Build history of the part. All positions in model axes, mm. A direction names the side the tool comes from. Give positions to 0.01 mm unless a question says otherwise; leave off trailing zeros. Write each loop counter-clockwise with the first axis right and the second up, starting at its lowest first coordinate (ties: lowest second). Pieces come first, ordered by that corner, then holes. Notation, with made-up numbers: (8.5, 81.5) -> (12.5, 81.5) arc R25 cw to (12.5, 100.5) -> close; hole circle Ø3 at (40, 64.5). An arc over 180 degrees is marked (long way). Put each result on its own line as item: value. Start each with the question number.
Item 1: Drill centre lines: line 1 along X through (y, z) = (-3.2, 5); line 2 along Z through (x, y) = (0, -6); line 3 along X through (y, z) = (-4, -4). Where is each one in solid material? Low to high.
Item 2: Two-plate mould, pull along Z, no slides. Class faces 3 (the flat face through (-3, 0, 3)), 4 (the cylindrical face through (-0.29, -2.46, 11.3)), 5 (the conical face through (-7.09, -11.74, 31.91)): pulls with the +Z half, pulls with the -Z half, needs draft (parallel to the pull), parting line crosses it, or undercut.
Item 3: Slice it at A-A, the plane y = -11. List the corners of the cut face in (x, z).
Item 4: Flat gauge pins, fed straight in: pin 1 Ø2 at (x, z) = (-5, 8.66) entering from +Y; pin 2 Ø4 at (x, z) = (-12.5, 15.5) entering from +Y; pin 3 Ø3 at (y, z) = (-8, -7) entering from -X; pin 4 Ø2 at (y, z) = (-3.5, 5.5) entering from -X. Where does each tip first touch, or does it go through?
Item 5: Tool access for faces 1 (the cylindrical face through (-3.73, -6.08, 9.06)), 2 (the flat face through (-9, -5, -5)): list every direction of +Z, -Z, +X, -X, +Y, -Y with a clear straight run to the whole face (end or side of a thin tool).
```python
from build123d import *

# Parameters (mm, degrees)
CONG_1_R                = 1
ENL_V_MAT_EXTRU_1_REACH = 14
ESQUISSE2_R             = 3.25
ESQUISSE2_R_2           = 1.33
ESQUISSE2_R_3           = 2
CHANFREIN1_SIZE         = 2
ESQUISSE3_R             = 1.33
ENL_V_MAT_EXTRU_2_DEPTH = 5


with BuildPart() as part:
    # Esquisse1 → Révolution1 (revolve)
    with BuildSketch(Plane.XY):
        Polygon((14, -5), (37.5, -5), (32.5, -12), (0, -12), (0, 0), (14, 0), align=None)
    revolve(axis=Axis((0, 0, 0), (0, 1, 0)))

    # Congé1
    cong_1_edges = [part.edges().sort_by_distance(p)[0] for p in [
        (-37.5, -5, 0),
        (-14, -5, 0),
        (-14, 0, 0),
    ]]
    fillet(cong_1_edges, radius=CONG_1_R)

    # Esquisse2 → Enlèv. mat.-Extru.1 (cut, up to next)
    with BuildSketch(Plane.XZ.offset(12), mode=Mode.PRIVATE) as enl_v_mat_extru_1_sk1:
        Circle(ESQUISSE2_R)
    enl_v_mat_extru_1_tool1 = extrude(enl_v_mat_extru_1_sk1.sketch, amount=-ENL_V_MAT_EXTRU_1_REACH, mode=Mode.PRIVATE) & part.part
    add(enl_v_mat_extru_1_tool1.solids().sort_by_distance((0, -12, 0))[0], mode=Mode.SUBTRACT)
    # Esquisse2 → Enlèv. mat.-Extru.1 (cut, up to next)
    with BuildSketch(Plane.XZ.offset(12), mode=Mode.PRIVATE) as enl_v_mat_extru_1_sk2:
        with Locations((10, 0)):
            Circle(ESQUISSE2_R_2)
    enl_v_mat_extru_1_tool2 = extrude(enl_v_mat_extru_1_sk2.sketch, amount=-ENL_V_MAT_EXTRU_1_REACH, mode=Mode.PRIVATE) & part.part
    add(enl_v_mat_extru_1_tool2.solids().sort_by_distance((10, -12, 0))[0], mode=Mode.SUBTRACT)
    # Esquisse2 → Enlèv. mat.-Extru.1 (cut, up to next)
    with BuildSketch(Plane.XZ.offset(12), mode=Mode.PRIVATE) as enl_v_mat_extru_1_sk3:
        with Locations((-5, -8.660254038)):
            Circle(ESQUISSE2_R_2)
    enl_v_mat_extru_1_tool3 = extrude(enl_v_mat_extru_1_sk3.sketch, amount=-ENL_V_MAT_EXTRU_1_REACH, mode=Mode.PRIVATE) & part.part
    add(enl_v_mat_extru_1_tool3.solids().sort_by_distance((-5, -12, -8.660254))[0], mode=Mode.SUBTRACT)
    # Esquisse2 → Enlèv. mat.-Extru.1 (cut, up to next)
    with BuildSketch(Plane.XZ.offset(12), mode=Mode.PRIVATE) as enl_v_mat_extru_1_sk4:
        with Locations((-5, 8.660254038)):
            Circle(ESQUISSE2_R_2)
    enl_v_mat_extru_1_tool4 = extrude(enl_v_mat_extru_1_sk4.sketch, amount=-ENL_V_MAT_EXTRU_1_REACH, mode=Mode.PRIVATE) & part.part
    add(enl_v_mat_extru_1_tool4.solids().sort_by_distance((-5, -12, 8.660254))[0], mode=Mode.SUBTRACT)
    # Esquisse2 → Enlèv. mat.-Extru.1 (cut, up to next)
    with BuildSketch(Plane.XZ.offset(12), mode=Mode.PRIVATE) as enl_v_mat_extru_1_sk5:
        with Locations((-8.5, 14.722431864)):
            Circle(ESQUISSE2_R_3)
    enl_v_mat_extru_1_tool5 = extrude(enl_v_mat_extru_1_sk5.sketch, amount=-ENL_V_MAT_EXTRU_1_REACH, mode=Mode.PRIVATE) & part.part
    add(enl_v_mat_extru_1_tool5.solids().sort_by_distance((-8.5, -12, 14.722432))[0], mode=Mode.SUBTRACT)

    # Chanfrein1
    chanfrein1_edges = [part.edges().sort_by_distance(p)[0] for p in [
        (-3.25, -12, 0),
    ]]
    chamfer(chanfrein1_edges, length=CHANFREIN1_SIZE)

    # Esquisse3 → Enlèv. mat.-Extru.2 (cut)
    with BuildSketch(Plane(origin=(0, 0, 0), x_dir=(1, 0, 0), z_dir=(0, 1, 0))):
        with Locations((8.660254038, 5)):
            Circle(ESQUISSE3_R)
        with Locations((8.660254038, -5)):
            Circle(ESQUISSE3_R)
        with Locations((-8.660254038, -5)):
            Circle(ESQUISSE3_R)
        with Locations((0, -10)):
            Circle(ESQUISSE3_R)
        with Locations((0, 10)):
            Circle(ESQUISSE3_R)
        with Locations((-8.660254038, 5)):
            Circle(ESQUISSE3_R)
    extrude(amount=-ENL_V_MAT_EXTRU_2_DEPTH, mode=Mode.SUBTRACT)


solid = part.part
```
Values follow:
1. line 1: -13.08 to -9.99, -7.33 to 7.33, 9.99 to 13.08
1. line 2: -36.56 to -3.25, 3.25 to 36.56
1. line 3: -13.42 to -9.54, -7.78 to 7.78, 9.54 to 13.42
2. face 3: needs draft
2. face 4: undercut
2. face 5: parting line crosses it
3. outline: circle Ø66.43 at (0, 0); hole circle Ø4 at (-8.5, 14.72); hole circle Ø2.66 at (-5, -8.66); hole circle Ø2.66 at (-5, 8.66); hole circle Ø8.5 at (0, 0); hole circle Ø2.66 at (10, 0)
4. pin 1: through
4. pin 2: y = -5
4. pin 3: x = -35.79
4. pin 4: x = -13.26
5. face 1: +Y, -Y
5. face 2: +Y
